```python
from build123d import *

# Parameters (mm, degrees)
BOSS_EXTRUDE1_DEPTH = 44.45
SKETCH3_R           = 1.5875
CUT_EXTRUDE1_DEPTH  = 25.4
CUT_EXTRUDE2_DEPTH  = 25.4


with BuildPart() as part:
    # Sketch1 → Boss-Extrude1 (new body)
    with BuildSketch(Plane(origin=(0, 0, 0), x_dir=(0, 0, -1), z_dir=(1, 0, 0))):
        Polygon((0, 19.05), (0, 0), (25.4, 0), (25.4, 3.175), (3.175, 3.175), (3.175, 19.05), align=None)
    extrude(amount=BOSS_EXTRUDE1_DEPTH)

    # Sketch3 → Cut-Extrude1 (cut)
    with BuildSketch(Plane(origin=(0, 0, -3.175), x_dir=(-1, 0, 0), z_dir=(0, 0, -1))):
        with Locations(Location((-38.225, 11.1125, 0), (0, 0, 90))):
            Circle(SKETCH3_R)
        with Locations(Location((-6.225, 11.1125, 0), (0, 0, 90))):
            Circle(SKETCH3_R)
    extrude(amount=-CUT_EXTRUDE1_DEPTH, mode=Mode.SUBTRACT)

    # Sketch4 → Cut-Extrude2 (cut)
    with BuildSketch(Plane(origin=(0, 3.175, 0), x_dir=(1, 0, 0), z_dir=(0, 1, 0))):
        with BuildLine():
            ThreePointArc((37.07765, 14.2875), (34.925, 16.44015), (32.77235, 14.2875))
            Line((32.77235, 14.2875), (34.925, 14.2875))
            Line((34.925, 14.2875), (37.07765, 14.2875))
        make_face()
        with BuildLine():
            Line((34.925, 14.2875), (32.77235, 14.2875))
            ThreePointArc((32.77235, 14.2875), (34.925, 12.13485), (37.07765, 14.2875))
            Line((37.07765, 14.2875), (34.925, 14.2875))
        make_face()
        with BuildLine():
            Line((7.37235, 14.2875), (9.525, 14.2875))
            Line((9.525, 14.2875), (11.67765, 14.2875))
            ThreePointArc((11.67765, 14.2875), (9.525, 16.44015), (7.37235, 14.2875))
        make_face()
        with BuildLine():
            Line((11.67765, 14.2875), (9.525, 14.2875))
            Line((9.525, 14.2875), (7.37235, 14.2875))
            ThreePointArc((7.37235, 14.2875), (9.525, 12.13485), (11.67765, 14.2875))
        make_face()
    extrude(amount=-CUT_EXTRUDE2_DEPTH, mode=Mode.SUBTRACT)


solid = part.part
```
The model under review builds one solid part; all positions refer to its coordinate system, in mm. A direction names the side the tool comes from. Round coordinates to 2 decimals unless told otherwise and drop trailing zeros. Loops run counter-clockwise (first coordinate to the right, second up) from the corner with the lowest first, then second, coordinate; pieces in that order, holes last.
1) The part is to be moulded in two halves that separate along X. For faces 3 (the face through (22, 10, 0)), 4 (the face through (0, 3, -8)), 5 (the face through (8.532, 1.61, -16.197)), say which applies: pulls with the +X half, pulls with the -X half, needs draft (parallel to the pull), parting line crosses it, or undercut.
Values follow:
face 3: needs draft
face 4: pulls with the -X half
face 5: undercut
2) Consider section C-C on x = 22. State the section outline as (y, z) points (3 decimals).
Values follow:
outline: (0, -25.4) - (3.175, -25.4) - (3.175, -3.175) - (19.05, -3.175) - (19.05, 0) - (0, 0) - close
3) Consider section B-B on z = -12.75. State the section outline as (x, y) points (3 decimals).
Values follow:
outline: (0, 0) - (8.018, 0) - (8.018, 3.175) - (0, 3.175) - close; (11.032, 0) - (33.418, 0) - (33.418, 3.175) - (11.032, 3.175) - close; (36.432, 0) - (44.45, 0) - (44.45, 3.175) - (36.432, 3.175) - close
4) Consider section D-D on y = 4.75. State the section outline as (x, z) points (3 decimals), then the cut area to 3 significant figures.
Values follow:
outline: (0, -3.175) - (44.45, -3.175) - (44.45, 0) - (0, 0) - close
area: 141 mm2
5) Consider section A-A on y = 10.25. State the section outline as (x, z) points (3 decimals), then the cut area to 3 significant figures.
Values follow:
outline: (0, -3.175) - (4.892, -3.175) - (4.892, 0) - (0, 0) - close; (7.558, -3.175) - (36.892, -3.175) - (36.892, 0) - (7.558, 0) - close; (39.558, -3.175) - (44.45, -3.175) - (44.45, 0) - (39.558, 0) - close
area: 124 mm2
6) Clearance check with flat-ended pins moving along their axes: P1, Ø5, axis at x = 27, z = -6, coming from the +Y side (3 decimals); P2, Ø1.5, axis at x = 17, y = 15.5, coming from the -Z side (3 decimals). State where each tip first meets the part, or that it passes through.
Values follow:
P1: stops at y = 3.175
P2: stops at z = -3.175
7) Tool access review of faces 1 (the face through (22, 3.175, -14)), 2 (the face through (44.45, 3, -8)): name each direction out of +Z, -Z, +X, -X, +Y, -Y from which nothing blocks a thin tool from reaching the whole face with its end or side.
Values follow:
face 1: -Z, +X, -X, +Y
face 2: +Z, -Z, +X, +Y, -Y
8) Wall thickness on line 1 along X through (y, z) = (1, -16); line 2 along Y through (x, z) = (40, -19) (3 decimals); line 3 along Z through (x, y) = (29, 16.25) (3 decimals): over which ranges is each line inside the solid? List them lowest first.
Values follow:
line 1: x = 0 to 8.22, 10.83 to 33.62, 36.23 to 44.45
line 2: y = 0 to 3.175
line 3: z = -3.175 to 0
